For this review, use the dimensioned drawing (mm, ordinates from the lowest corner) and the shaded views. A direction names the side the tool comes from. Give positions to 0.01 mm unless a question says otherwise; leave off trailing zeros. Order: outer loops, then holes, each group sorted by start corner. A loop starts at its lowest first (then second) coordinate and runs counter-clockwise, first axis right, second up. Notation, with made-up numbers: (-24, -24.5) -> (29, -24.5) arc R34 ccw to (29, 14.5) -> close; hole circle Ø2 at (48.5, 39). An arc over 180 degrees is marked (long way). Return JSON: item names as keys, results as strings.
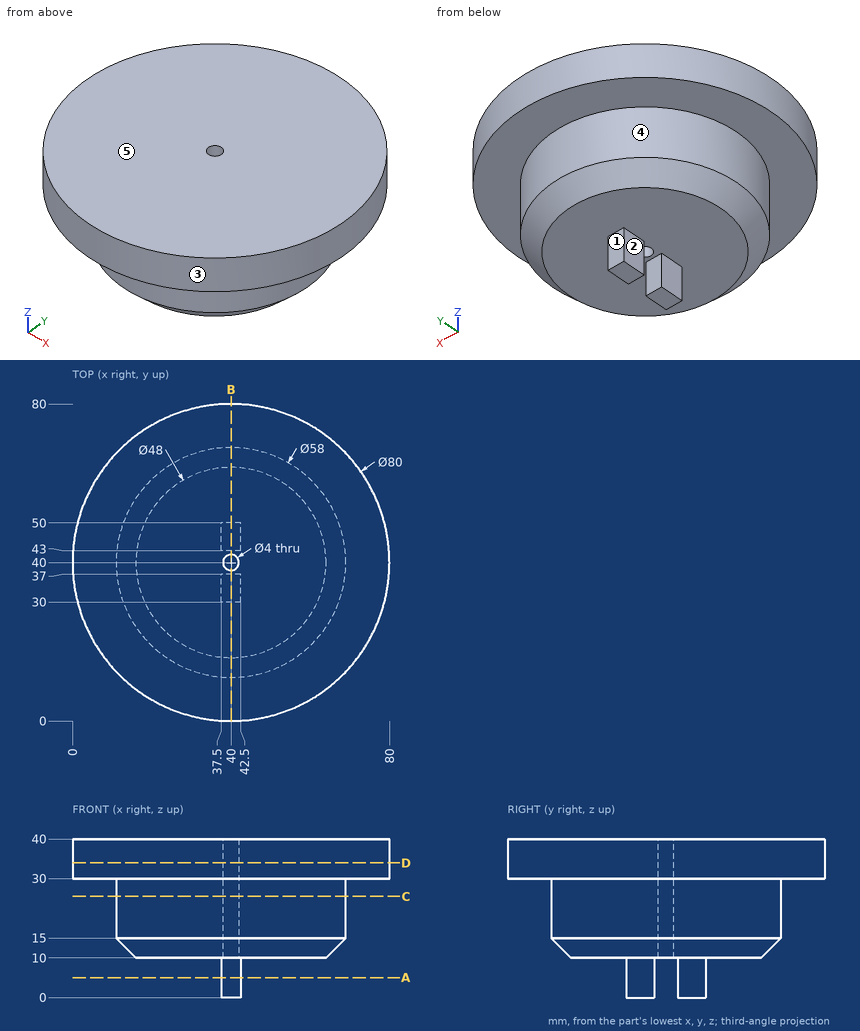
Item 1: For pin 1 (2 mm diameter, centred on x = 17, z = 22.5, fed in from +Y); pin 2 (1.5 mm diameter, centred on x = 39, z = 7.5, fed in from +Y); pin 3 (1 mm diameter, centred on x = 29, z = 20, fed in from +Y), all flat-tipped, find the tip position at first contact; note any pin that passes through.
Result set:
{"pin 1": "stops at y = 58.89", "pin 2": "stops at y = 50", "pin 3": "stops at y = 67.03"}
Item 2: Add section B-B (x = 40). Give the boundary of the cut face in (y, z).
Result set:
{"outline": "(0, 30) -> (11, 30) -> (11, 15) -> (16, 10) -> (30, 10) -> (30, 0) -> (37, 0) -> (37, 10) -> (38, 10) -> (38, 40) -> (0, 40) -> close; (42, 10) -> (43, 10) -> (43, 0) -> (50, 0) -> (50, 10) -> (64, 10) -> (69, 15) -> (69, 30) -> (80, 30) -> (80, 40) -> (42, 40) -> close"}
Item 3: Wall thickness on L1, parallel to Z at x = 73.5, y = 22.5; L2, parallel to Y at x = 40, z = 32.5; L3, parallel to Z at x = 31.5, y = 44.5: over which ranges is each line inside the solid? List them lowest first. Write a range as [from, to].
Result set:
{"L1": "z = [30, 40]", "L2": "y = [0, 38], [42, 80]", "L3": "z = [10, 40]"}
Item 4: Machinability: for the marked faces 1, 2, 3, 4 and 5, which of the approach directions +Z, -Z, +X, -X, +Y, -Y give a long, thin tool a straight path to every point of the face, cutting with its end or side? Answer none if there is none.
Result set:
{"face 1": "-Z, +X, -X, +Y", "face 2": "-Z, -X, +Y, -Y", "face 3": "+Z, -Z", "face 4": "-Z", "face 5": "+Z, +X, -X, +Y, -Y"}
Item 5: Add section A-A (z = 5). Give the boundary of the cut face in (x, y), plus the area to 3 significant figures.
Result set:
{"outline": "(37.5, 30) -> (42.5, 30) -> (42.5, 37) -> (37.5, 37) -> close; (37.5, 43) -> (42.5, 43) -> (42.5, 50) -> (37.5, 50) -> close", "area": "70.0 mm^2"}
Item 6: Add section C-C (z = 25.5). Give the boundary of the cut face in (x, y).
Result set:
{"outline": "circle Ø58 at (40, 40); hole circle Ø4 at (40, 40)"}
Item 7: Add section D-D (z = 34). Give the boundary of the cut face in (x, y).
Result set:
{"outline": "circle Ø80 at (40, 40); hole circle Ø4 at (40, 40)"}
